Autodesk Inventor part; units mm, degrees
ref_plane "YZ Plane" through (0, 0, 0) normal (1, 0, 0) x (0, 1, 0)
ref_plane "XZ Plane" through (0, 0, 0) normal (0, 1, 0) x (-1, 0, 0)
ref_plane "XY Plane" through (0, 0, 0) normal (0, 0, 1) x (1, 0, 0)
sketch "Sketch1" plane through (0, 0, 0) normal (1, 0, 0) x (0, 1, 0)
  arc A0 (4.3225, -9.9221) -> (5.9696, -5.6989) centre (-2.06, -5) ccw
  arc A1 (5.9244, -3.8989) -> (4.3225, -0.0779) centre (-2.06, -5) ccw
  arc A2 (-5.9696, -5.6989) -> (-4.3225, -9.9221) centre (2.06, -5) ccw
  arc A3 (-4.3225, -0.0779) -> (-5.9244, -3.8989) centre (2.06, -5) ccw
  line L0 (4.1641, 0) -> (-4.1641, 0)
  line L1 (-4.1641, -10) -> (4.1641, -10)
  line L2 (6, -10) -> (6, 0)
  line L3 (6, 0) -> (-6, 0)
  line L4 (-6, 0) -> (-6, -10)
  line L5 (-6, -10) -> (-7.27, -10)
  line L6 (-7.27, -10) -> (-7.27, 1.27)
  line L7 (6, -10) -> (7.27, -10)
  line L8 (6, 0) -> (6, 1.27) construction
  line L9 (6, 1.27) -> (-7.27, 1.27)
  line L10 (7.27, -10) -> (7.27, 1.27)
  line L11 (7.27, 1.27) -> (6, 1.27)
  point P0 (0, 0)
  dimension "d0" = 1.27
  dimension "d1" = 1.27
  dimension "d2" = 1.27
extrude "Extrusion1" add sketch "Sketch1" along normal blind 11.1125
sketch "Sketch2" plane through (0, 7.27, 1.27) normal (0, 1, 0) x (1, 0, 0)
  line L0 (11.1125, 11.27) -> (11.1125, 0)
  line L1 (0, 11.27) -> (11.1125, 11.27)
  line L2 (0, 0) -> (0, 11.27)
  line L3 (11.1125, 11.27) -> (3.175, 11.27)
  line L4 (0, 11.27) -> (11.1125, 11.27)
  line L5 (3.175, 11.27) -> (3.175, 10)
  line L6 (3.175, 10) -> (11.1125, 10)
  point P0 (0, 1.27)
  dimension "d5" = 7.9375
  dimension "d6" = 1.27
extrude "Extrusion2" add sketch "Sketch2" along normal blind 6.35
fillet "Fillet1" radius 3.9688 1 edges at (11.1125, 13.62, -9.365)
fillet "Fillet2" radius 3.9688 1 edges at (3.175, 13.62, -9.365)
sketch "Sketch3" plane through (3.175, 7.27, -8.73) normal (0, 0, 1) x (1, 0, 0)
  arc A0 (7.9375, 2.3812) -> (0, 2.3813) centre (3.9688, 2.3812) ccw
  line L0 (0, 0) -> (0, 2.3813)
  line L1 (7.9375, 0) -> (0, 0)
  line L2 (7.9375, 0) -> (7.9375, 2.3812)
  circle A1 centre (3.9688, 2.3812) radius 1.27
  point P0 (-3.175, -7.27)
  dimension "d11" = 2.54
hole "Hole1" at (7.1438, 9.6513, -8.73) direction (0, 0, -1) diameter 2.54 end through all
sketch "Sketch4" plane through (0, -7.27, -10) normal (0, -1, 0) x (1, 0, 0)
  line L0 (0, 0) -> (0, 11.27)
  line L1 (0, 0) -> (11.1125, 0)
  line L2 (11.1125, 11.27) -> (11.1125, 0)
  line L3 (0, 11.27) -> (11.1125, 11.27)
  line L4 (0, 0) -> (11.1125, 0)
  line L5 (11.1125, 0) -> (3.175, 0)
  line L6 (11.1125, 1.27) -> (3.175, 1.27)
  line L7 (3.175, 0) -> (3.175, 1.27)
  line L8 (3.175, 1.27) -> (11.1125, 1.27)
  line L9 (11.1125, 1.27) -> (11.1125, 0)
  line L10 (11.1125, 1.27) -> (11.1125, 0)
  point P0 (0, 10)
  dimension "d19" = 7.9375
  dimension "d20" = 1.27
extrude "Extrusion3" add sketch "Sketch4" along normal blind 6.35 contours L7 L6 L2 L1
fillet "Fillet3" radius 3.9688 1 edges at (3.175, -13.62, -9.365)
fillet "Fillet4" radius 3.9688 1 edges at (11.1125, -13.62, -9.365)
sketch "Sketch5" plane through (3.175, -7.27, -8.73) normal (0, 0, 1) x (1, 0, 0)
  arc A0 (0, -2.3813) -> (7.9375, -2.3813) centre (3.9688, -2.3813) ccw
  line L0 (7.9375, 0) -> (7.9375, -2.3813)
  line L1 (0, 0) -> (7.9375, 0)
  line L2 (0, 0) -> (0, -2.3813)
  circle A1 centre (3.9688, -2.3813) radius 1.27
  point P0 (-3.175, 7.27)
  dimension "d25" = 2.54
hole "Hole2" at (7.1438, -9.6513, -8.73) direction (0, 0, -1) diameter 2.54 end through all
fillet "Fillet5" radius 1.27 1 edges at (5.5563, -7.27, 1.27)
fillet "Fillet6" radius 1.27 1 edges at (5.5563, 7.27, 1.27)
properties part number "Mount" material "PAEK Plastic"
Design review of the part built by this model. Coordinates are the model's own, in mm. A direction names the side the tool comes from. Give positions to 0.01 mm unless a question says otherwise; leave off trailing zeros. Order: outer loops, then holes, each group sorted by start corner. A loop starts at its lowest first (then second) coordinate and runs counter-clockwise, first axis right, second up. Notation, with made-up numbers: (58.5, -22.75) - (78.5, -22.75) arc R21 cw to (78.5, -10.75) - close; hole circle Ø6 at (-10, 78.25). An arc over 180 degrees is marked (long way). Use CSV: the item, a comma, the result in double quotes. Start each with the question number.
Q1. For P1, Ø0.6, axis at y = 8, z = -9.5, coming from the -X side (3 decimals); P2, Ø1.9, axis at x = 7.5, y = -12, coming from the +Z side; P3, Ø3.5, axis at x = 6, y = -2, coming from the -Z side, all flat-tipped, find the tip position at first contact; note any pin that passes through.
Q2. For line 1 (Y direction, x = 5.5, z = -2); line 2 (Z direction, x = 8, y = 5.5); line 3 (Z direction, x = 7.75, y = 7.5), list the stretches that pass through material, from the lowest coordinate up.
Q3. Machinability: for faces 1 (the face through (3.175, -8, -9)), 2 (the face through (7.2, -11.1, -8.73)), 3 (the face through (7.1, 11.1, -8.73)), 4 (the face through (5, 0, 0)), which of the approach directions +Z, -Z, +X, -X, +Y, -Y give a long, thin tool a straight path to every point of the face, cutting with its end or side? Answer none if there is none.
Q4. Take a section at C-C (y = -9.25). State the section outline as (x, z) points (1 decimal), and give its area (3 significant figures).
Q5. Take a section at B-B (x = 1). State the section outline as (y, z) points, and give its area (3 significant figures).
Q6. Take a section at A-A (z = -2.25). State the section outline as (x, y) points, and give its area (3 significant figures).
Q7. Take a section at D-D (x = 6.75). State the section outline as (y, z) points, and give its area (3 significant figures).
Q8. Draft analysis for pull direction Y (two halves, no side actions). For faces 5 (the face through (4.37, 12.49, -9.36)), 6 (the face through (6.3, 10.6, -9.4)), 7 (the face through (11.112, 0, 0.3)), state which applies: pulls with the +Y half, pulls with the -Y half, needs draft (parallel to the pull), parting line crosses it, or undercut.
Calculated:
1,P1,"stops at x = 3.175"
1,P2,"stops at z = -8.73"
1,P3,"stops at z = 0"
2,line 1,"y = -7.27 to -6, 6 to 7.27"
2,line 2,"z = 0 to 1.27"
2,line 3,"z = -10 to -8.73"
3,face 1,"+Z, -Z, -X, -Y"
3,face 2,"+Z, +X, -X, -Y"
3,face 3,"+Z, +X, -X, +Y"
3,face 4,"-Z, +X, -X"
4,outline,"(3.2, -10) - (5.9, -10) - (5.9, -8.7) - (3.2, -8.7) - close; (8.3, -10) - (11.1, -10) - (11.1, -8.7) - (8.3, -8.7) - close"
4,area,"7.02 mm²"
5,outline,"(-7.27, -10) - (-6, -10) - (-6, 0) - (6, 0) - (6, -10) - (7.27, -10) - (7.27, 0) arc R1.27 ccw to (6, 1.27) - (-6, 1.27) arc R1.27 ccw to (-7.27, 0) - close"
5,area,"43.2 mm²"
6,outline,"(0, -7.27) - (11.11, -7.27) - (11.11, -6) - (0, -6) - close; (0, 6) - (11.11, 6) - (11.11, 7.27) - (0, 7.27) - close"
6,area,"28.2 mm²"
7,outline,"(-13.6, -10) - (-10.86, -10) - (-10.86, -8.73) - (-13.6, -8.73) - close; (-8.44, -10) - (-6, -10) - (-6, 0) - (6, 0) - (6, -10) - (8.44, -10) - (8.44, -8.73) - (7.27, -8.73) - (7.27, 0) arc R1.27 ccw to (6, 1.27) - (-6, 1.27) arc R1.27 ccw to (-7.27, 0) - (-7.27, -8.73) - (-8.44, -8.73) - close; (10.86, -10) - (13.6, -10) - (13.6, -8.73) - (10.86, -8.73) - close"
7,area,"53.1 mm²"
8,face 5,"pulls with the +Y half"
8,face 6,"undercut"
8,face 7,"needs draft"
